Work out the finished part from the listing and answer in its coordinate system (mm). A direction names the side the tool comes from. Give positions to 0.01 mm unless a question says otherwise; leave off trailing zeros. Loops run counter-clockwise (first coordinate to the right, second up) from the corner with the lowest first, then second, coordinate; pieces in that order, holes last. Notation, with made-up numbers: (71.5, -10.75) - (105.5, -10.75) arc R18 cw to (105.5, 11.25) - close; hole circle Ø10 at (25, 47). An arc over 180 degrees is marked (long way). One line per item, written item: value.
from build123d import *

# Parameters (mm, degrees)
F0_W     = 914.4
F0_H     = 2120.9
F1_DEPTH = 50.8
F2_R     = 25.4
F3_DEPTH = 50.801
F4_W     = 34.790657
F4_H     = 464.079693
F5_DEPTH = 254


with BuildPart() as f1:
    # F0 (on Front) → F1 (new body)
    with BuildSketch(Plane.XZ):
        Rectangle(F0_W, F0_H)
    extrude(amount=F1_DEPTH)

    # F2 (on face) → F3 (cut, through all)
    with BuildSketch(Plane.XZ.offset(50.8)):
        with Locations((406.4, 247.65)):
            Circle(F2_R)
        with Locations((406.4, 146.05)):
            Circle(F2_R)
    extrude(amount=-F3_DEPTH, mode=Mode.SUBTRACT)

    # F4 (on face) → F5 (cut)
    with BuildSketch(Plane.YZ.offset(457.2)):
        with Locations((-25.352478, 163.164123)):
            Rectangle(F4_W, F4_H)
    extrude(amount=-F5_DEPTH, mode=Mode.SUBTRACT)


solid = f1.part
1. A flat-ended cylindrical pin translates along its axis: pin 1 Ø17.5 at (y, z) = (-22, 238) entering from +X. Find the tip coordinate at first contact, or state that the pin passes through.
Output:
pin 1: stops at x = 203.2
2. Section A-A (z = 247.65) is taken. Write down the section's boundary in (x, y).
Output:
outline: (-457.2, -50.8) - (381, -50.8) - (381, -42.75) - (203.2, -42.75) - (203.2, -7.96) - (381, -7.96) - (381, 0) - (-457.2, 0) - close; (431.8, -50.8) - (457.2, -50.8) - (457.2, -42.75) - (431.8, -42.75) - close; (431.8, -7.96) - (457.2, -7.96) - (457.2, 0) - (431.8, 0) - close
3. Find the intervals of material crossed by line 1 along Z through (x, y) = (406.4, -46.5); line 2 along Z through (x, y) = (358.5, -32); line 3 along X through (y, z) = (-4, 146), in increasing order.
Output:
line 1: z = -1060.45 to 120.65, 171.45 to 222.25, 273.05 to 1060.45
line 2: z = -1060.45 to -68.88, 395.2 to 1060.45
line 3: x = -457.2 to 381, 431.8 to 457.2
4. For faces 5 (the flat face through (332, -26, 395.204)), 6 (the cylindrical face through (430.627, -4.034, 255.279)), determine the directions among +Z, -Z, +X, -X, +Y, -Y from which every point of the face is accessible in a straight line to the end or side of a thin tool.
Output:
face 5: +X
face 6: +Y, -Y
5. Section C-C (y = -31.5) is taken. Write down the section's boundary in (x, z).
Output:
outline: (-457.2, -1060.45) - (457.2, -1060.45) - (457.2, -68.88) - (203.2, -68.88) - (203.2, 395.2) - (457.2, 395.2) - (457.2, 1060.45) - (-457.2, 1060.45) - close
6. The mould has two halves that part along Y. Classify faces 1 (the flat face through (-6, -50.8, 15)), 2 (the flat face through (332, -26, -68.876)), 3 (the flat face through (-6, -25, 1060.45)), 4 (the flat face through (332, -7.957, 160)): released by +Y, released by -Y, zero draft, split by the parting line, or undercut.
Output:
face 1: released by -Y
face 2: undercut
face 3: zero draft
face 4: undercut
7. Section D-D (x = 406.4) is taken. Write down the section's boundary in (y, z).
Output:
outline: (-50.8, -1060.45) - (0, -1060.45) - (0, 120.65) - (-7.96, 120.65) - (-7.96, -68.88) - (-42.75, -68.88) - (-42.75, 120.65) - (-50.8, 120.65) - close; (-50.8, 171.45) - (-42.75, 171.45) - (-42.75, 222.25) - (-50.8, 222.25) - close; (-50.8, 273.05) - (-42.75, 273.05) - (-42.75, 395.2) - (-7.96, 395.2) - (-7.96, 273.05) - (0, 273.05) - (0, 1060.45) - (-50.8, 1060.45) - close; (-7.96, 171.45) - (0, 171.45) - (0, 222.25) - (-7.96, 222.25) - close
8. Section B-B (x = 232) is taken. Write down the section's boundary in (y, z), and give its area (3 significant figures).
Output:
outline: (-50.8, -1060.45) - (0, -1060.45) - (0, 1060.45) - (-50.8, 1060.45) - close; hole (-42.75, -68.88) - (-7.96, -68.88) - (-7.96, 395.2) - (-42.75, 395.2) - close
area: 91,600 mm²
